Work out the finished part from the listing and answer in its coordinate system (mm). A direction names the side the tool comes from. Coordinates: 2 decimals unless noted, no trailing zeros. Order: outer loops, then holes, each group sorted by start corner. A loop starts at its lowest first (then second) coordinate and runs counter-clockwise, first axis right, second up. Notation, with made-up numbers: M -30,-38 L -2,-38 A14 ccw -2,-24 Z; hole C -30,73.5 d6. An arc over 180 degrees is marked long. Use a Markdown table: item, result.
from build123d import *

# Parameters (mm, degrees)
SKETCH1_W            = 47.8
SKETCH1_H            = 47.8
SKETCH1_W_2          = 40.2
SKETCH1_H_2          = 40.2
BOSS_EXTRUDE1_DEPTH  = 5
CUT_EXTRUDE4_REACH   = 55.675
SKETCH6_R            = 1.35
CUT_EXTRUDE5_REACH   = 55.675
SKETCH7_R            = 1.35
SKETCH8_R            = 1.35
CUT_EXTRUDE6_DEPTH   = 54.675413366
SKETCH11_W           = 5
SKETCH11_H           = 28
SKETCH11_W_2         = 47.8
SKETCH11_H_2         = 47.8
SKETCH11_R           = 1.65
BOSS_EXTRUDE8_DEPTH  = 8
CUT_EXTRUDE7_DEPTH   = 105.393965343
SKETCH12_R           = 1.35
BOSS_EXTRUDE9_DEPTH  = 5
BOSS_EXTRUDE10_START = -2
SKETCH12_3_R         = 8.5
BOSS_EXTRUDE10_DEPTH = 3


with BuildPart() as part:
    # Sketch1 → Boss-Extrude1 (new body)
    with BuildSketch(Plane(origin=(0, 0, 0), x_dir=(1, 0, 0), z_dir=(0, 1, 0))):
        Rectangle(SKETCH1_W, SKETCH1_H)
        Rectangle(SKETCH1_W_2, SKETCH1_H_2, mode=Mode.SUBTRACT)
    extrude(amount=BOSS_EXTRUDE1_DEPTH)

    # Sketch6 → Cut-Extrude4 (cut, up to next)
    with BuildSketch(Plane(origin=(0, 0, -23.9), x_dir=(-1, 0, 0), z_dir=(0, 0, -1)), mode=Mode.PRIVATE) as cut_extrude4_sk1:
        with Locations((-12.9, 3)):
            Circle(SKETCH6_R)
    cut_extrude4_tool1 = extrude(cut_extrude4_sk1.sketch, amount=-CUT_EXTRUDE4_REACH, mode=Mode.PRIVATE) & part.part
    # Sketch6 → Cut-Extrude4 (cut, up to next)
    with BuildSketch(Plane(origin=(0, 0, -23.9), x_dir=(-1, 0, 0), z_dir=(0, 0, -1)), mode=Mode.PRIVATE) as cut_extrude4_sk2:
        with Locations((12.9, 3)):
            Circle(SKETCH6_R)
    cut_extrude4_tool2 = extrude(cut_extrude4_sk2.sketch, amount=-CUT_EXTRUDE4_REACH, mode=Mode.PRIVATE) & part.part
    add(cut_extrude4_tool1.solids().sort_by_distance((12.9, 3, -23.9))[0], mode=Mode.SUBTRACT)
    add(cut_extrude4_tool2.solids().sort_by_distance((-12.9, 3, -23.9))[0], mode=Mode.SUBTRACT)

    # Sketch7 → Cut-Extrude5 (cut, up to next)
    with BuildSketch(Plane.XY.offset(23.9), mode=Mode.PRIVATE) as cut_extrude5_sk1:
        with Locations((9.4, 2.5)):
            Circle(SKETCH7_R)
    cut_extrude5_tool1 = extrude(cut_extrude5_sk1.sketch, amount=-CUT_EXTRUDE5_REACH, mode=Mode.PRIVATE) & part.part
    # Sketch7 → Cut-Extrude5 (cut, up to next)
    with BuildSketch(Plane.XY.offset(23.9), mode=Mode.PRIVATE) as cut_extrude5_sk2:
        with Locations((-5.6, 2.5)):
            Circle(SKETCH7_R)
    cut_extrude5_tool2 = extrude(cut_extrude5_sk2.sketch, amount=-CUT_EXTRUDE5_REACH, mode=Mode.PRIVATE) & part.part
    add(cut_extrude5_tool1.solids().sort_by_distance((9.4, 2.5, 23.9))[0], mode=Mode.SUBTRACT)
    add(cut_extrude5_tool2.solids().sort_by_distance((-5.6, 2.5, 23.9))[0], mode=Mode.SUBTRACT)

    # Sketch8 → Cut-Extrude6 (cut, through all)
    with BuildSketch(Plane(origin=(23.9, 0, 0), x_dir=(0, 0, -1), z_dir=(1, 0, 0))):
        with Locations((-9.9, 3)):
            Circle(SKETCH8_R)
        with Locations(Location((9.9, 3, 0), (0, 0, 180))):
            Circle(SKETCH8_R)
    extrude(amount=-CUT_EXTRUDE6_DEPTH, mode=Mode.SUBTRACT)

    # Sketch11 → Boss-Extrude8 (add)
    # profile 1 of 3: a face of its own
    with BuildSketch(Plane(origin=(0, 0, 0), x_dir=(1, 0, 0), z_dir=(0, 1, 0))):
        Polygon((73.9, -21.4), (68.9, -21.4), (68.9, -49.4), (-23.9, -23.9), (23.9, -23.9), (23.9, 23.9), align=None)
    # profile 2 of 3: a face of its own
    with BuildSketch(Plane(origin=(0, 0, 0), x_dir=(1, 0, 0), z_dir=(0, 1, 0))):
        with Locations((71.4, -35.4)):
            Rectangle(SKETCH11_W, SKETCH11_H)
    # profile 3 of 3: a face of its own
    with BuildSketch(Plane(origin=(0, 0, 0), x_dir=(1, 0, 0), z_dir=(0, 1, 0))):
        Rectangle(SKETCH11_W_2, SKETCH11_H_2)
        with Locations(Location((-16, -16, 0), (0, 0, 270))):
            Circle(SKETCH11_R, mode=Mode.SUBTRACT)
        with Locations(Location((16, -16, 0), (0, 0, 270))):
            Circle(SKETCH11_R, mode=Mode.SUBTRACT)
        with Locations(Location((16, 16, 0), (0, 0, 270))):
            Circle(SKETCH11_R, mode=Mode.SUBTRACT)
        with Locations(Location((-16, 16, 0), (0, 0, 270))):
            Circle(SKETCH11_R, mode=Mode.SUBTRACT)
    extrude(amount=-BOSS_EXTRUDE8_DEPTH)

    # Sketch13 → Cut-Extrude7 (cut, through all)
    with BuildSketch(Plane.XY.offset(49.4)):
        Polygon((73.9, -3.587183479), (64.114380232, -3.587183479), (28.73812358, 1.78739259), (73.9, 1.78739259), align=None)
    extrude(amount=-CUT_EXTRUDE7_DEPTH, mode=Mode.SUBTRACT)

    # Sketch12 → Boss-Extrude9 (add)
    # profile 1 of 2: a face of its own
    with BuildSketch(Plane(origin=(73.9, 0, 0), x_dir=(0, 0, -1), z_dir=(1, 0, 0))):
        with BuildLine():
            Line((-23.099667517, 0), (-21.4, 0))
            Line((-21.4, 0), (-21.4, 24.412816521))
            Line((-21.4, 24.412816521), (-49.4, 24.412816521))
            Line((-49.4, 24.412816521), (-49.4, 0))
            Line((-49.4, 0), (-47.700332483, 0))
            ThreePointArc((-47.700332483, 0), (-46.9, 0.262816521), (-46.099667517, 0))
            Line((-46.099667517, 0), (-39.386947717, 0))
            ThreePointArc((-39.386947717, 0), (-41.719336712, 19.599136977), (-24.25, 10.412816521))
            ThreePointArc((-24.25, 10.412816521), (-26.213679544, 4.093479809), (-31.413052283, 0))
            Line((-31.413052283, 0), (-24.700332483, 0))
            ThreePointArc((-24.700332483, 0), (-23.9, 0.262816521), (-23.099667517, 0))
        make_face()
        with Locations((-46.9, 21.912816521)):
            Circle(SKETCH12_R, mode=Mode.SUBTRACT)
        with Locations((-23.9, 21.912816521)):
            Circle(SKETCH12_R, mode=Mode.SUBTRACT)
    # profile 2 of 2: a face of its own
    with BuildSketch(Plane(origin=(73.9, 0, 0), x_dir=(0, 0, -1), z_dir=(1, 0, 0))):
        with BuildLine():
            Line((-49.4, -3.587183479), (-21.4, -3.587183479))
            Line((-21.4, -3.587183479), (-21.4, 0))
            Line((-21.4, 0), (-23.099667517, 0))
            ThreePointArc((-23.099667517, 0), (-22.695228476, -0.478064793), (-22.55, -1.087183479))
            ThreePointArc((-22.55, -1.087183479), (-24.509118686, -2.291955003), (-24.700332483, 0))
            Line((-24.700332483, 0), (-31.413052283, 0))
            ThreePointArc((-31.413052283, 0), (-35.4, -0.737183479), (-39.386947717, 0))
            Line((-39.386947717, 0), (-46.099667517, 0))
            ThreePointArc((-46.099667517, 0), (-45.695228476, -0.478064793), (-45.55, -1.087183479))
            ThreePointArc((-45.55, -1.087183479), (-47.509118686, -2.291955003), (-47.700332483, 0))
            Line((-47.700332483, 0), (-49.4, 0))
            Line((-49.4, 0), (-49.4, -3.587183479))
        make_face()
    extrude(amount=-BOSS_EXTRUDE9_DEPTH)

    # Sketch12_3 → Boss-Extrude10 (add)
    # profile 1 of 2: a face of its own
    with BuildSketch(Plane(origin=(73.9, 0, 0), x_dir=(0, 0, -1), z_dir=(1, 0, 0)).offset(BOSS_EXTRUDE10_START)):
        with BuildLine():
            Line((-39.386947717, 0), (-31.413052283, 0))
            ThreePointArc((-31.413052283, 0), (-26.213679544, 4.093479809), (-24.25, 10.412816521))
            ThreePointArc((-24.25, 10.412816521), (-41.719336712, 19.599136977), (-39.386947717, 0))
        make_face()
        with Locations((-35.4, 10.412816521)):
            Circle(SKETCH12_3_R, mode=Mode.SUBTRACT)
    # profile 2 of 2: a face of its own
    with BuildSketch(Plane(origin=(73.9, 0, 0), x_dir=(0, 0, -1), z_dir=(1, 0, 0)).offset(BOSS_EXTRUDE10_START)):
        with BuildLine():
            ThreePointArc((-39.386947717, 0), (-35.4, -0.737183479), (-31.413052283, 0))
            Line((-31.413052283, 0), (-39.386947717, 0))
        make_face()
    extrude(amount=-BOSS_EXTRUDE10_DEPTH)


solid = part.part
1. For faces 5 (the face through (23.9, 2, 0)), 6 (the face through (70.42, 16.16, 41.66)), 7 (the face through (0, 0, 0)), 8 (the face through (9.11, 1.18, 22.03)), 9 (the face through (15.368, -3.944, -14.476)), determine the directions among +Z, -Z, +X, -X, +Y, -Y from which every point of the face is accessible in a straight line to the end or side of a thin tool.
Answers below:
| item | result |
|---|---|
| face 5 | +Z, -Z, +Y |
| face 6 | +X, -X |
| face 7 | +Y |
| face 8 | +Z |
| face 9 | +Y, -Y |
2. Section B-B on y = 14.5 is taken. Determine the outline of the cut face in (x, z).
Answers below:
| item | result |
|---|---|
| outline | M 68.9,21.4 L 73.9,21.4 L 73.9,25.03 L 71.9,25.03 L 71.9,27.95 L 68.9,27.95 Z; M 68.9,42.85 L 71.9,42.85 L 71.9,45.77 L 73.9,45.77 L 73.9,49.4 L 68.9,49.4 Z |
3. For a pull along Z with two mould halves and no side action, classify faces 1 (the face through (71, 10, 21.4)), 2 (the face through (71.44, 23.25, 47.08)), 3 (the face through (-4.353, 1.983, 22.027)), 4 (the face through (0, 2, 23.9)) as +Z half, -Z half, draft (parallel to the pull), parting line (faces both ways), or undercut.
Answers below:
| item | result |
|---|---|
| face 1 | -Z half |
| face 2 | undercut |
| face 3 | draft |
| face 4 | +Z half |
4. Section C-C on z = 35.4 is taken. Determine the outline of the cut face in (x, y), then the cut area to 3 significant figures.
Answers below:
| item | result |
|---|---|
| outline | M 17.95,-8 L 73.9,-8 L 73.9,-0.74 L 71.9,-0.74 L 71.9,1.91 L 68.9,1.91 L 68.9,-3.59 L 64.11,-3.59 L 40.5,0 L 17.95,0 Z; M 68.9,18.91 L 71.9,18.91 L 71.9,21.56 L 73.9,21.56 L 73.9,24.41 L 68.9,24.41 Z |
| area | 415 mm² |
5. Section A-A on x = 9.4 is taken. Determine the outline of the cut face in (y, z).
Answers below:
| item | result |
|---|---|
| outline | M -8,-23.9 L 5,-23.9 L 5,-20.1 L 0,-20.1 L 0,20.1 L 1.15,20.1 L 1.15,23.9 L 0,23.9 L 0,33.05 L -8,33.05 Z; M 3.85,20.1 L 5,20.1 L 5,23.9 L 3.85,23.9 Z |
6. Find the intervals of material crossed by probe 1 along Y at (x, z) = (71, 46.9); probe 2 along Y at (x, z) = (-21.8, -9.9); probe 3 along Y at (x, z) = (72, 35), in increasing order.
Answers below:
| item | result |
|---|---|
| probe 1 | -8 to -2.44, 0.26 to 20.56, 23.26 to 24.41 |
| probe 2 | -8 to 1.65, 4.35 to 5 |
| probe 3 | -8 to -0.73, 21.56 to 24.41 |
7. Section D-D on z = -16 is taken. Determine the outline of the cut face in (x, y), then the cut area to 3 significant figures.
Answers below:
| item | result |
|---|---|
| outline | M -23.9,-8 L -17.65,-8 L -17.65,0 L -20.1,0 L -20.1,5 L -23.9,5 Z; M -14.35,-8 L 14.35,-8 L 14.35,0 L -14.35,0 Z; M 17.65,-8 L 32.62,-8 L 32.62,0 L 23.9,0 L 23.9,5 L 20.1,5 L 20.1,0 L 17.65,0 Z |
| area | 437 mm² |
8. Flat-ended cylindrical pins translate along their axes: P1, Ø20, axis at x = -8.5, z = 6, coming from the +Y side; P2, Ø3, axis at y = 10.5, z = 28, coming from the +X side; P3, Ø5.5, axis at y = 3.5, z = 4.5, coming from the +X side. Find the tip coordinate at first contact, or state that the pin passes through.
Answers below:
| item | result |
|---|---|
| P1 | y = 0 |
| P2 | x = 71.9 |
| P3 | x = 23.9 |
